Geometry check sheet. Reference: the model listing, model coordinates, mm. Face numbers are marked on the shaded views. A direction names the side the tool comes from. Round coordinates to 2 decimals unless told otherwise and drop trailing zeros. Order: outer loops, then holes, each group sorted by start corner. A loop starts at its lowest first (then second) coordinate and runs counter-clockwise, first axis right, second up. Notation, with made-up numbers: (-23.5, 69) - (17.5, 69) arc R21 ccw to (17.5, 80) - close; hole circle Ø4 at (73, 0). An arc over 180 degrees is marked (long way). Return JSON: item names as keys, results as strings. Group by question number.
Q1. Draft check along Z on the marked faces 1, 2 and 3. Enter one of: pulls with the +Z half, pulls with the -Z half, needs draft (parallel to the pull), parting line crosses it, or undercut.
Q2. Material ranges on line 1 along X through (y, z) = (26.5, 0); line 2 along X through (y, z) = (11.75, 33), recorded low to high.
Q3. Tool access check on the marked faces 4 and 5. Record the directions out of +Z, -Z, +X, -X, +Y, -Y that give a thin tool (end or side, any length) a straight path to the whole face; none if there is none.
Q4. Sectioned sample at C-C, the plane x = 52.4. Record the cut outline in (y, z), then the cut area to 3 significant figures.
Q5. Sectioned sample at A-A, the plane x = -18. Record the cut outline in (y, z), then the cut area to 3 significant figures.
Q6. Gauge pin test, flat ends, axial feed: pin 1 Ø1.1 at (y, z) = (0.5, -3.5) entering from +X; pin 2 Ø1.3 at (x, z) = (52.5, -1.5) entering from -Y; pin 3 Ø0.6 at (x, y) = (-51, 27.5) entering from +Z. Record the tip position at first contact, or that the pin passes through.
Q7. Sectioned sample at B-B, the plane z = -15. Record the cut outline in (x, y).
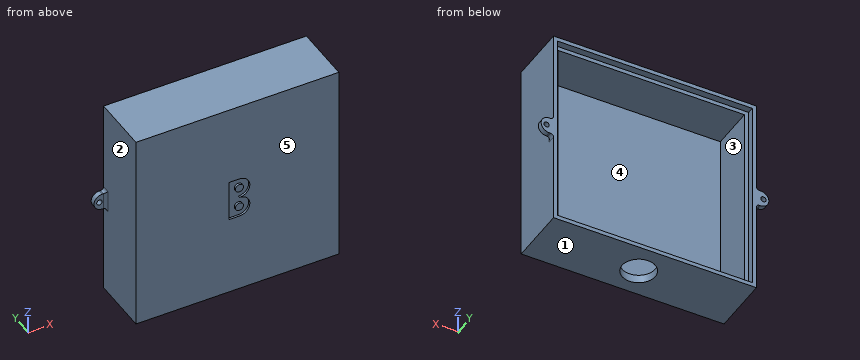
```python
from build123d import *

# Parameters (mm, degrees)
SKETCH1_W           = 98
SKETCH1_H           = 98
BOSS_EXTRUDE1_DEPTH = 30
SKETCH2_W           = 94
SKETCH2_H           = 94
CUT_EXTRUDE1_DEPTH  = 5
SKETCH3_W           = 90
SKETCH3_H           = 90
CUT_EXTRUDE2_DEPTH  = 21
SKETCH4_W           = 98
SKETCH4_H           = 98
SKETCH4_W_2         = 94
SKETCH4_H_2         = 94
CUT_EXTRUDE3_DEPTH  = 1.8
SKETCH5_R           = 1.3
BOSS_EXTRUDE2_DEPTH = 2.5
FILLET1_R           = 1.5
FILLET2_R           = 1.5
CUT_EXTRUDE4_REACH  = 100
SKETCH6_R           = 8
SKETCH7_R           = 1.968352886
CUT_EXTRUDE5_DEPTH  = 1


with BuildPart() as part:
    # Sketch1 → Boss-Extrude1 (new body)
    with BuildSketch(Plane(origin=(0, 0, 0), x_dir=(1, 0, 0), z_dir=(0, 1, 0))):
        Rectangle(SKETCH1_W, SKETCH1_H)
    extrude(amount=BOSS_EXTRUDE1_DEPTH)

    # Sketch2 → Cut-Extrude1 (cut)
    with BuildSketch(Plane(origin=(0, 30, 0), x_dir=(1, 0, 0), z_dir=(0, 1, 0))):
        Rectangle(SKETCH2_W, SKETCH2_H)
    extrude(amount=-CUT_EXTRUDE1_DEPTH, mode=Mode.SUBTRACT)

    # Sketch3 → Cut-Extrude2 (cut)
    with BuildSketch(Plane(origin=(0, 25, 0), x_dir=(1, 0, 0), z_dir=(0, 1, 0))):
        Rectangle(SKETCH3_W, SKETCH3_H)
    extrude(amount=-CUT_EXTRUDE2_DEPTH, mode=Mode.SUBTRACT)

    # Sketch4 → Cut-Extrude3 (cut)
    with BuildSketch(Plane(origin=(0, 30, 0), x_dir=(1, 0, 0), z_dir=(0, 1, 0))):
        Rectangle(SKETCH4_W, SKETCH4_H)
        Rectangle(SKETCH4_W_2, SKETCH4_H_2, mode=Mode.SUBTRACT)
    extrude(amount=-CUT_EXTRUDE3_DEPTH, mode=Mode.SUBTRACT)

    # Sketch5 → Boss-Extrude2 (add)
    with BuildSketch(Plane(origin=(0, 28.2, 0), x_dir=(1, 0, 0), z_dir=(0, 1, 0))):
        with BuildLine():
            Line((-49, 4), (-51, 4))
            ThreePointArc((-51, 4), (-55, 0), (-51, -4))
            Line((-51, -4), (-49, -4))
            Line((-49, -4), (-49, 4))
        make_face()
        with Locations((-52.4, 0)):
            Circle(SKETCH5_R, mode=Mode.SUBTRACT)
        with BuildLine():
            Line((49, 4), (49, -4))
            Line((49, -4), (51, -4))
            ThreePointArc((51, -4), (55, 0), (51, 4))
            Line((51, 4), (49, 4))
        make_face()
        with Locations((52.4, 0)):
            Circle(SKETCH5_R, mode=Mode.SUBTRACT)
    extrude(amount=-BOSS_EXTRUDE2_DEPTH)

    # Fillet1
    fillet1_edges = [part.edges().sort_by_distance(p)[0] for p in [
        (-49, 25.7, 0),
        (-49, 26.95, -4),
        (-49, 26.95, 4),
    ]]
    fillet(fillet1_edges, radius=FILLET1_R)

    # Fillet2
    fillet2_edges = [part.edges().sort_by_distance(p)[0] for p in [
        (49, 26.95, -4),
        (49, 25.7, 0),
        (49, 26.95, 4),
    ]]
    fillet(fillet2_edges, radius=FILLET2_R)

    # Sketch6 → Cut-Extrude4 (cut, up to next)
    with BuildSketch(Plane(origin=(0, 0, -49), x_dir=(-1, 0, 0), z_dir=(0, 0, -1)), mode=Mode.PRIVATE) as cut_extrude4_sk1:
        with Locations((0, 14)):
            Circle(SKETCH6_R)
    cut_extrude4_tool1 = extrude(cut_extrude4_sk1.sketch, amount=-CUT_EXTRUDE4_REACH, mode=Mode.PRIVATE) & part.part
    add(cut_extrude4_tool1.solids().sort_by_distance((0, 14, -49))[0], mode=Mode.SUBTRACT)

    # Sketch7 → Cut-Extrude5 (cut)
    with BuildSketch(Plane.XZ):
        with BuildLine():
            Line((-4, -10), (-1, -10))
            Line((-1, -10), (1, -10))
            ThreePointArc((1, -10), (6, -5), (1, 0))
            ThreePointArc((1, 0), (6, 5), (1, 10))
            Line((1, 10), (-4, 10))
            Line((-4, 10), (-4, -10))
        make_face()
        with Locations((1, 5)):
            Circle(SKETCH7_R, mode=Mode.SUBTRACT)
        with Locations((1, -5)):
            Circle(SKETCH7_R, mode=Mode.SUBTRACT)
    extrude(amount=-CUT_EXTRUDE5_DEPTH, mode=Mode.SUBTRACT)


solid = part.part
```
Reply:
{
 "1": {"face 1": "pulls with the -Z half", "face 2": "needs draft", "face 3": "undercut"},
 "2": {"line 1": "-55 to -53.7, -51.1 to -47, 47 to 51.1, 53.7 to 55", "line 2": "-49 to -45, 45 to 49"},
 "3": {"face 4": "+Y", "face 5": "+Z, -Z, +X, -X, -Y"},
 "4": {"outline": "(25.7, -3.75) - (28.2, -3.75) - (28.2, -1.3) - (25.7, -1.3) - close; (25.7, 1.3) - (28.2, 1.3) - (28.2, 3.75) - (25.7, 3.75) - close", "area": "12.2 mm^2"},
 "5": {"outline": "(0, -49) - (28.2, -49) - (28.2, -47) - (25, -47) - (25, -45) - (4, -45) - (4, 45) - (25, 45) - (25, 47) - (28.2, 47) - (28.2, 49) - (0, 49) - close", "area": "573 mm^2"},
 "6": {"pin 1": "x = 49", "pin 2": "y = 25.7", "pin 3": "z = 4"},
 "7": {"outline": "(-49, 0) - (49, 0) - (49, 28.2) - (47, 28.2) - (47, 25) - (45, 25) - (45, 4) - (-45, 4) - (-45, 25) - (-47, 25) - (-47, 28.2) - (-49, 28.2) - close"}
}
